Check sheet for the modelled part. Datum: model origin and axes. Units: mm. A direction names the side the tool comes from. Round coordinates to 2 decimals unless told otherwise and drop trailing zeros. Write each loop counter-clockwise with the first axis right and the second up, starting at its lowest first coordinate (ties: lowest second). Pieces come first, ordered by that corner, then holes. Notation, with made-up numbers: (3.5, 6.5) - (12.5, 6.5) arc R11 ccw to (12.5, 18.5) - close; hole circle Ø10 at (43, 54). An arc over 180 degrees is marked (long way). Use one line per item in the form item = value. Start each with the question number.
1) Section check A-A (z = 14). Record the boundary of the cut face in (x, y).
2) Gauge pin test, flat ends, axial feed: P1, Ø0.5, axis at y = 33.5, z = 5, coming from the -X side; P2, Ø0.5, axis at y = -34, z = 6, coming from the +X side; P3, Ø2, axis at y = 20.5, z = 34.5, coming from the +X side. Record the tip position at first contact, or that the pin passes through.
3) Draft check along Y on faces 1 (the face through (-27.85, -8.77, 0.89)), 2 (the face through (0, -34, 5)), 3 (the face through (6.54, 32.87, 4.98)), 4 (the face through (3.348, 33.521, 6.313)). Enter one of: +Y half, -Y half, draft (parallel to the pull), parting line (faces both ways), or undercut.
4) Set-up check for faces 5 (the face through (32.87, -6.54, 4.98)), 6 (the face through (4.036, -30.736, 21.106)), 7 (the face through (-32.87, 6.54, 4.98)): record each of +Z, -Z, +X, -X, +Y, -Y from which the full face is reachable in a straight line by a thin tool's end or side.
5) Scan lines: probe 1 along X at (y, z) = (0, 1); probe 2 along X at (y, z) = (0, 40.4); probe 3 along Z at (x, y) = (24, -19). Record each from-to range of solid material in increasing order.
from build123d import *

# Parameters (mm, degrees)
SKETCH003_W        = 2
SKETCH003_H        = 10
GROOVE_ANGLE       = 78.75
POLARPATTERN_COUNT = 4


with BuildPart() as part:
    # Sketch002 → Revolution002 (revolve)
    with BuildSketch(Plane.XZ):
        Polygon((-32.8, 46.066667), (-29.2, 46.066667), (-29.2, 44.266667), (-31, 42.466667), (-31, 42.066667), (-30.198, 41.264667), (-30.198, 40.064667), (-31, 39.10888), (-31, 3.6), (-29.2, 1.8), (-29.2, 0), (-32.8, 0), (-32.8, 2.7), (-34.6, 4.5), (-34.6, 5.4), (-32.8, 7.2), (-32.8, 44.266667), align=None)
    revolve(axis=Axis((0, 0, 0), (0, 0, 1)))

    # Sketch003 → Groove (revolve, cut)
    with BuildSketch(Plane.XZ):
        with Locations((-33.8, 5)):
            Rectangle(SKETCH003_W, SKETCH003_H)
    groove = revolve(axis=Axis((0, 0, 0), (0, 0, 1)), revolution_arc=GROOVE_ANGLE, mode=Mode.SUBTRACT)

    # PolarPattern: Groove ×4 about axis
    polarpattern_axis = Axis((0, 0, 0), (0, 0, 1))
    for i in range(1, POLARPATTERN_COUNT):
        add(groove.rotate(polarpattern_axis, i * 360 / POLARPATTERN_COUNT), mode=Mode.SUBTRACT)


solid = part.part
Results are:
q1.outline = circle Ø65.6 at (0, 0); hole circle Ø62 at (0, 0)
q2.P1 = 0
q2.P2 = 0
q2.P3 = 26.37
q3.face_1 = undercut
q3.face_2 = draft
q3.face_3 = undercut
q3.face_4 = +Y half
q4.face_5 = +Z, -Z, -Y
q4.face_6 = none
q4.face_7 = +Z, -Z, +Y
q5.probe_1 = -32.8 to -29.2, 29.2 to 32.8
q5.probe_2 = -32.8 to -30.2, 30.2 to 32.8
q5.probe_3 = 0 to 3.21, 39.57 to 41.68, 42.86 to 46.07
